from build123d import *

# Parameters (mm, degrees)
SKETCH1_W           = 30
SKETCH1_H           = 42
BOSS_EXTRUDE1_DEPTH = 5
SKETCH2_R           = 1.125
CUT_EXTRUDE1_DEPTH  = 37.959437225
CHAMFER1_SIZE       = 4.367642811
CHAMFER1_SIZE_2     = 12
CHAMFER2_SIZE       = 12
CHAMFER2_SIZE_2     = 4.367642811


with BuildPart() as part:
    # Sketch1 → Boss-Extrude1 (new body)
    with BuildSketch(Plane(origin=(0, 0, 0), x_dir=(1, 0, 0), z_dir=(0, 1, 0))):
        Rectangle(SKETCH1_W, SKETCH1_H)
    extrude(amount=BOSS_EXTRUDE1_DEPTH)

    # Sketch2 → Cut-Extrude1 (cut, through all)
    with BuildSketch(Plane(origin=(15, 0, 0), x_dir=(0, 0, -1), z_dir=(1, 0, 0))):
        with Locations((-19, 3)):
            Circle(SKETCH2_R)
        with Locations((-16.285714286, 3)):
            Circle(SKETCH2_R)
        with Locations((-13.571428571, 3)):
            Circle(SKETCH2_R)
        with Locations((-10.857142857, 3)):
            Circle(SKETCH2_R)
        with Locations((-8.142857143, 3)):
            Circle(SKETCH2_R)
        with Locations((-5.428571429, 3)):
            Circle(SKETCH2_R)
        with Locations((-2.714285714, 3)):
            Circle(SKETCH2_R)
        with Locations((0, 3)):
            Circle(SKETCH2_R)
        with Locations((2.714285714, 3)):
            Circle(SKETCH2_R)
        with Locations((5.428571429, 3)):
            Circle(SKETCH2_R)
        with Locations((8.142857143, 3)):
            Circle(SKETCH2_R)
        with Locations((10.857142857, 3)):
            Circle(SKETCH2_R)
        with Locations((13.571428571, 3)):
            Circle(SKETCH2_R)
        with Locations((16.285714286, 3)):
            Circle(SKETCH2_R)
        with Locations((19, 3)):
            Circle(SKETCH2_R)
    extrude(amount=-CUT_EXTRUDE1_DEPTH, mode=Mode.SUBTRACT)

    # Chamfer1
    # the kernel refuses this chamfer: 12, 4.367642811 mm, written as the material it takes off along each edge
    with BuildSketch(Plane(origin=(15, 5, 52.130336791), x_dir=(0.09904090225204926, -0.9950833631817486, 0), z_dir=(0, 0, -1))) as chamfer1_piece_1:
        Polygon((CHAMFER1_SIZE * 0.995083363226, CHAMFER1_SIZE * 0.0990409022565), (-CHAMFER1_SIZE_2 * 0.099040902252, CHAMFER1_SIZE_2 * 0.995083363182), (0, 0), align=None)
    extrude(amount=104.260673581, mode=Mode.SUBTRACT)

    # Chamfer2
    # the kernel refuses this chamfer: 12, 4.367642811 mm, written as the material it takes off along each edge
    with BuildSketch(Plane(origin=(-15, 5, -52.130336791), x_dir=(0.9999130865277315, 0.013184058198645937, 0), z_dir=(0, 0, 1))) as chamfer2_piece_1:
        Polygon((CHAMFER2_SIZE * 0.999913086528, -CHAMFER2_SIZE * 0.0131840581986), (-CHAMFER2_SIZE_2 * 0.0131840581992, -CHAMFER2_SIZE_2 * 0.999913086572), (0, 0), align=None)
    extrude(amount=104.260673581, mode=Mode.SUBTRACT)


solid = part.part
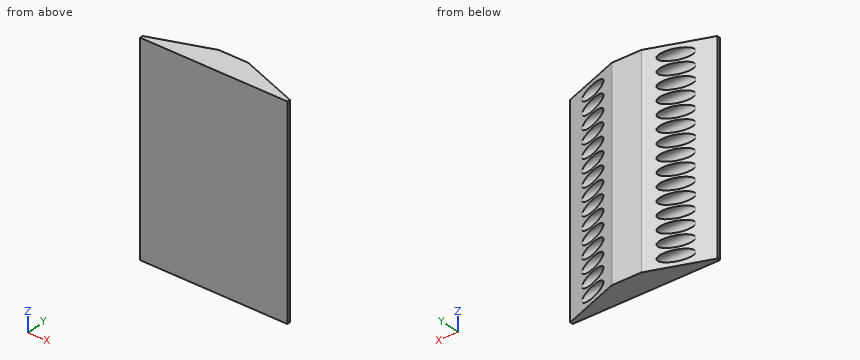
Can you work these out from the model? Positions are in its coordinate system, mm. Give positions to 0.01 mm unless a question says otherwise; leave off trailing zeros. Loops run counter-clockwise (first coordinate to the right, second up) from the corner with the lowest first, then second, coordinate; pieces in that order, holes last. Notation, with made-up numbers: M 46.5,52.5 L 103.5,52.5 A12 cw 103.5,74.5 Z; hole C 66.25,10 d1. An arc over 180 degrees is marked long. One line per item, written item: value. Start each with the question number.
1) If we section it at D-D, the plane z = 2.5: Write out the boundary of the cut face in (x, y), and give its area (3 significant figures).
2) I'm going to push a flat-ended pin straight in: pin 1 (2 mm diameter, centred on y = 3, z = 16.29, fed in from -X). Where does the tip first touch, or does it pass through?
3) If we section it at A-A, the plane z = 13: Write out the boundary of the cut face in (x, y), and give its area (3 significant figures).
4) If we section it at B-B, the plane x = -3.75: Give the number of separate pieces and of enclosed holes in the cut face, and give its area (3 significant figures).
5) If I drill on line 1 (Y direction, x = 0, z = 11); line 2 (Y direction, x = -2, z = -2); line 3 (Y direction, x = 12, z = -6), over which ranges is the centre line in solid material (lowest first)? Write a range as [from, to].
Completed:
1. outline: M -15,0 L 15,0 L 15,0.63 L 11.53,1.9 L -11.53,1.9 L -15,0.63 Z; M -5.46,4.1 L 5.46,4.1 L 3,5 L -3,5 Z
1. area: 60.1 mm^2
2. pin 1: passes through
3. outline: M -15,0 L 15,0 L 15,0.63 L 11.16,2.03 L -11.16,2.03 L -15,0.63 Z; M -5.83,3.97 L 5.83,3.97 L 3,5 L -3,5 Z
3. area: 64.7 mm^2
4. separate pieces: 1
4. enclosed holes: 15
4. area: 139 mm^2
5. line 1: y = [0, 1.88], [4.12, 5]
5. line 2: y = [0, 2.13], [3.87, 5]
5. line 3: y = [0, 1.72]
